from build123d import *

# Parameters (mm, degrees)
SKETCH2_R          = 2.5527
CUT_EXTRUDE1_DEPTH = 18.897183893


with BuildPart() as part:
    # Sketch1 → Revolve1 (revolve)
    with BuildSketch(Plane.XY):
        Polygon((-27.857278892, 8.0391), (-14.024094998, 8.0391), (-14.024094998, 25.4), (-9.960094998, 25.4), (-9.960094998, 36.83), (-18.295757287, 36.83), (-27.857278892, 17.801339222), align=None)
    revolve(axis=Axis((0, 0, 0), (-1, 0, 0)))

    # Sketch2 → Cut-Extrude1 (cut, through all)
    with BuildSketch(Plane(origin=(-9.960094998, 0, 0), x_dir=(0, 0, -1), z_dir=(1, 0, 0))):
        with Locations((35.086604814, -8.389036369)):
            Circle(SKETCH2_R)
        with Locations((1.050672613, -7.874611544)):
            Circle(SKETCH2_R)
        with Locations((18.860257121, 44.244090147)):
            Circle(SKETCH2_R)
        with Locations((46.093533365, 23.822092726)):
            Circle(SKETCH2_R)
        with Locations((-8.977761775, 24.654449577)):
            Circle(SKETCH2_R)
    extrude(amount=-CUT_EXTRUDE1_DEPTH, mode=Mode.SUBTRACT)


solid = part.part
Work out the finished part from the listing and answer in its coordinate system (mm). A direction names the side the tool comes from. Give positions to 0.01 mm unless a question says otherwise; leave off trailing zeros. Loops run counter-clockwise (first coordinate to the right, second up) from the corner with the lowest first, then second, coordinate; pieces in that order, holes last. Notation, with made-up numbers: (70.25, 58.25) -> (78.25, 58.25) arc R18 ccw to (78.25, 79.25) -> close; hole circle Ø10 at (40.5, -19.5). An arc over 180 degrees is marked (long way). Use a Markdown table: item, result. Add a question column.
1. For faces 1 (the cylindrical face through (-17.326, 27.185, 9.31)), 2 (the flat face through (-14.024, 6, -6)), determine the directions among +Z, -Z, +X, -X, +Y, -Y from which every point of the face is accessible in a straight line to the end or side of a thin tool.
2. Flat-ended cylindrical pins translate along their axes: pin 1 Ø5 at (x, y) = (-13.5, 4) entering from +Z; pin 2 Ø14.5 at (y, z) = (0, 0) entering from -X; pin 3 Ø5 at (x, y) = (-20, -25) entering from +Z; pin 4 Ø1.5 at (y, z) = (10.5, -24) entering from -X. Find the tip coordinate at first contact, or state that the pin passes through.
3. Section B-B on x = -12 is taken. Determine the outline of the cut face in (y, z), and give its area (3 significant figures).
4. Determine the mould class of faces 3 (the conical face through (-27.39, -18.71, -0.82)), 4 (the cylindrical face through (-20.84, -10.41, -1.33)), 5 (the flat face through (-27.857, 8, 4)) for opening direction Y: released by +Y, released by -Y, zero draft, split by the parting line, or undercut.
5. Section A-A on y = 0 is taken. Determine the outline of the cut face in (x, z), and give its area (4 significant figures).
6. Find the intervals of material crossed by probe 1 along X at (y, z) = (0.5, 11); probe 2 along Y at (x, z) = (-11.5, 6); probe 3 along Y at (x, z) = (-24.25, -4.5), in increasing order.
Results below:
| question | item | result |
|---|---|---|
| 1 | face 1 | +X, -X |
| 1 | face 2 | +X |
| 2 | pin 1 | stops at z = 36.8 |
| 2 | pin 2 | passes through |
| 2 | pin 3 | stops at z = 28.63 |
| 2 | pin 4 | stops at x = -24.02 |
| 3 | outline | (-10.94, -35.17) arc R2.55 cw (long way) to (-6.15, -36.31) arc R36.83 ccw (long way) to start; hole (22.95, 10.88) arc R25.4 ccw (long way) to (24.57, 6.43) arc R2.55 ccw (long way) to start |
| 3 | area | 2,210 mm^2 |
| 4 | face 3 | split by the parting line |
| 4 | face 4 | undercut |
| 4 | face 5 | zero draft |
| 5 | outline | (-27.86, -17.8) -> (-18.3, -36.83) -> (-9.96, -36.83) -> (-9.96, -25.4) -> (-14.02, -25.4) -> (-14.02, -8.04) -> (-27.86, -8.04) -> close; (-27.86, 8.04) -> (-14.02, 8.04) -> (-14.02, 25.4) -> (-9.96, 25.4) -> (-9.96, 36.83) -> (-18.3, 36.83) -> (-27.86, 17.8) -> close |
| 5 | area | 707.5 mm^2 |
| 6 | probe 1 | x = -27.86 to -14.02 |
| 6 | probe 2 | y = -36.34 to -24.68, 24.68 to 36.34 |
| 6 | probe 3 | y = -24.57 to -6.66, 6.66 to 24.57 |
